Verification items for this drawing (mm, ordinates from the low corner). Coordinates: 2 decimals unless noted, no trailing zeros. Loops run counter-clockwise (first coordinate to the right, second up) from the corner with the lowest first, then second, coordinate; pieces in that order, holes last.
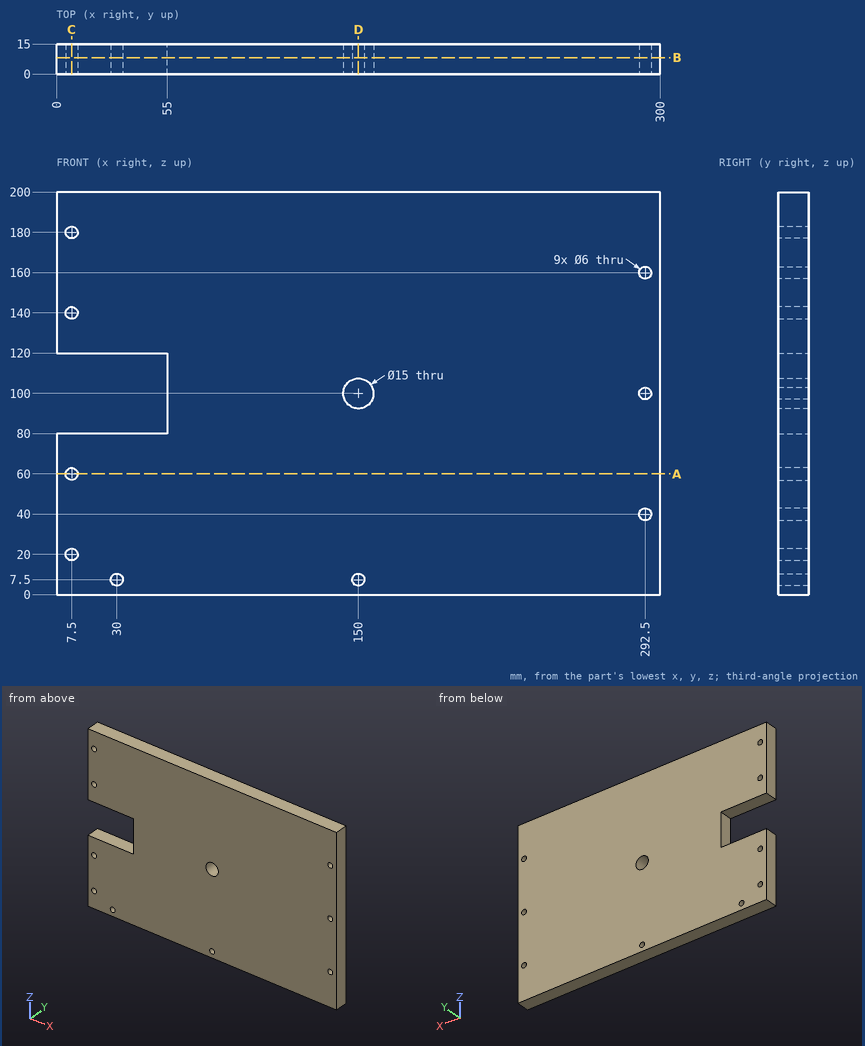
(1) Gauge pin test, flat end, axial feed: P1, Ø3.5, axis at x = 7.5, z = 140, coming from the +Y side. Record the tip position at first contact, or that the pin passes through.
(2) Section check A-A, the plane z = 60. Enter the section's corners in (x, y), plus the area to 3 significant figures.
(3) Section check C-C, the plane x = 7.5. Enter the section's corners in (y, z).
(4) Scan lines: line 1 along Z through (x, y) = (292.5, 4); line 2 along X through (y, z) = (9.75, 20); line 3 along X through (y, z) = (6.5, 7.5). Record each from-to range of solid material in increasing order.
(5) Section check B-B, the plane y = 8.25. Count the separate pieces of the cut face and the enclosed holes in it, plus the area to 3 significant figures.
(6) Section check D-D, the plane x = 150. Enter the section's corners in (y, z), plus the area to 4 significant figures.
Determined:
1. P1: passes through
2. outline: (0, 0) - (4.5, 0) - (4.5, 15) - (0, 15) - close; (10.5, 0) - (300, 0) - (300, 15) - (10.5, 15) - close
2. area: 4,410 mm2
3. outline: (0, 0) - (15, 0) - (15, 17) - (0, 17) - close; (0, 23) - (15, 23) - (15, 57) - (0, 57) - close; (0, 63) - (15, 63) - (15, 80) - (0, 80) - close; (0, 120) - (15, 120) - (15, 137) - (0, 137) - close; (0, 143) - (15, 143) - (15, 177) - (0, 177) - close; (0, 183) - (15, 183) - (15, 200) - (0, 200) - close
4. line 1: z = 0 to 37, 43 to 97, 103 to 157, 163 to 200
4. line 2: x = 0 to 4.5, 10.5 to 300
4. line 3: x = 0 to 27, 33 to 147, 153 to 300
5. separate pieces: 1
5. enclosed holes: 10
5. area: 57,400 mm2
6. outline: (0, 0) - (15, 0) - (15, 4.5) - (0, 4.5) - close; (0, 10.5) - (15, 10.5) - (15, 92.5) - (0, 92.5) - close; (0, 107.5) - (15, 107.5) - (15, 200) - (0, 200) - close
6. area: 2,685 mm2
